For this review, take the finished solid that the model builds, in its own axes (mm). A direction names the side the tool comes from. Give positions to 0.01 mm unless a question says otherwise; leave off trailing zeros. Order: outer loops, then holes, each group sorted by start corner. A loop starts at its lowest first (then second) coordinate and runs counter-clockwise, first axis right, second up. Notation, with made-up numbers: (72.5, 56.5) -> (106.5, 56.5) arc R27 ccw to (106.5, 91.5) -> close; hole circle Ø5 at (31, 72.25). An arc over 180 degrees is marked (long way). Return JSON: item names as keys, results as strings. Group by question number.
1) To check wall thickness, follow line 1 along X through (y, z) = (-79.6, 592.5); line 2 along Y through (x, z) = (20.5, 792); line 3 along X through (y, z) = (-1.5, 739). State the ranges of each line that lie inside material, in increasing order.
2) Insertion check: P1, Ø2, axis at y = -23, z = 789.5, coming from the +X side; P2, Ø8, axis at y = -65.5, z = 991, coming from the -X side; P3, Ø9, axis at x = -50, z = 592.5, coming from the -Y side. Each pin has a flat end and moves straight along its axis. Give the tip position at first contact, or say it passes through.
3) Add section A-A (x = 21). Give the boundary of the cut face in (y, z), then the cut area to 3 significant figures.
4) Add section B-B (z = 976.5). Give the boundary of the cut face in (x, y).
5) For faces 1 (the face through (-3, -1, 584)), 2 (the face through (-1, 82.55, 584)), 3 (the face through (3, 1, 584)), list the 3-axis set-ups (+Z, -Z, +X, -X, +Y, -Y) from which the entire face can be reached by the end or side of a thin tool; tool diameter is ignored.
6) Add section C-C (y = 34.5). Give the boundary of the cut face in (x, z).
7) The part is to be moulded in two halves that separate along Y. For faces 4 (the face through (0, 0, 1185)), 5 (the face through (40, 76.55, 584)), 6 (the face through (1, -82.55, 584)), say which applies: released by +Y, released by -Y, zero draft, split by the parting line, or undercut.
from build123d import *

# Parameters (mm, degrees)
BOSS_EXTRUDE1_DEPTH = 1185
SKETCH3_R           = 5
CUT_EXTRUDE2_DEPTH  = 20


with BuildPart() as part:
    # Sketch1 → Boss-Extrude1 (new body)
    with BuildSketch(Plane.XY):
        Polygon((3, -76.55), (76.2, -76.55), (76.2, -82.55), (-76.2, -82.55), (-76.2, -76.55), (-3, -76.55), (-3, 76.55), (-76.2, 76.55), (-76.2, 82.55), (76.2, 82.55), (76.2, 76.55), (3, 76.55), align=None)
    extrude(amount=BOSS_EXTRUDE1_DEPTH)

    # Sketch3 → Cut-Extrude2 (cut)
    with BuildSketch(Plane.XZ.offset(82.55)):
        with Locations(Location((-50, 592.5, 0), (0, 0, 270))):
            Circle(SKETCH3_R)
        with Locations(Location((50, 592.5, 0), (0, 0, 270))):
            Circle(SKETCH3_R)
    extrude(amount=-CUT_EXTRUDE2_DEPTH, mode=Mode.SUBTRACT)


solid = part.part
Evaluation:
{
 "1": {"line 1": "-76.2 to -55, -45 to 45, 55 to 76.2", "line 2": "-82.55 to -76.55, 76.55 to 82.55", "line 3": "-3 to 3"},
 "2": {"P1": "x = 3", "P2": "x = -3", "P3": "y = 76.55"},
 "3": {"outline": "(-82.55, 0) -> (-76.55, 0) -> (-76.55, 1185) -> (-82.55, 1185) -> close; (76.55, 0) -> (82.55, 0) -> (82.55, 1185) -> (76.55, 1185) -> close", "area": "14,200 mm^2"},
 "4": {"outline": "(-76.2, -82.55) -> (76.2, -82.55) -> (76.2, -76.55) -> (3, -76.55) -> (3, 76.55) -> (76.2, 76.55) -> (76.2, 82.55) -> (-76.2, 82.55) -> (-76.2, 76.55) -> (-3, 76.55) -> (-3, -76.55) -> (-76.2, -76.55) -> close"},
 "5": {"face 1": "+Z, -Z, -X", "face 2": "+Z, -Z, +X, -X, +Y", "face 3": "+Z, -Z, +X"},
 "6": {"outline": "(-3, 0) -> (3, 0) -> (3, 1185) -> (-3, 1185) -> close"},
 "7": {"face 4": "zero draft", "face 5": "undercut", "face 6": "released by -Y"}
}
